Read the model definition and answer for the solid it produces. Units are mm, in the model's axes. A direction names the side the tool comes from. Give positions to 0.01 mm unless a question says otherwise; leave off trailing zeros. Order: outer loops, then holes, each group sorted by start corner. A loop starts at its lowest first (then second) coordinate and runs counter-clockwise, first axis right, second up.
Item 1: A cutting plane is placed at A-A (x = 50). Write down the section's boundary in (y, z), plus the area to 3 significant figures.
Item 2: A cutting plane is placed at C-C (z = 12). Write down the section's boundary in (x, y), plus the area to 3 significant figures.
Item 3: A cutting plane is placed at D-D (z = 15.5). Write down the section's boundary in (x, y).
Item 4: Which of the six approach directions +Z, -Z, +X, -X, +Y, -Y give full straight-line access (tool end or side, diameter ignored) to faces 4 (the face through (57.594, 9.126, 2.281)), 5 (the face through (32.1, 4.06, 29.14)), 6 (the face through (28.813, 2.958, 24.961)), 7 (the face through (1.2, 10.03, 12.95)), 8 (the face through (53, 13, 20))?
Item 5: A cutting plane is placed at B-B (y = 2.5). Write down the section's boundary in (x, z), plus the area to 3 significant figures.
Item 6: The mould has two halves that part along Z. Classify faces 1 (the face through (30, 6, 1)), 2 (the face through (2.281, 9.126, 2.406)), 3 (the face through (38.3, 8.6, 23)): +Z half, -Z half, draft (parallel to the pull), parting line (faces both ways), or undercut.
Item 7: Given pin 1 Ø3 at (x, z) = (28.5, 29) entering from +Y; pin 2 Ø8 at (y, z) = (9, 1.5) entering from -X; pin 3 Ø2 at (x, z) = (44.5, 26.5) entering from -Y; pin 4 Ø6 at (x, z) = (27.5, 15) entering from +Y, each flat-ended and moving along its own axis, determine where each tip first touches the part or whether it passes through.
Item 8: Find the intervals of material crossed by line 1 along Z through (x, y) = (30.2, 4.15); line 2 along X through (y, z) = (11.5, 18.5); line 3 along X through (y, z) = (16.5, 9), in increasing order.
from build123d import *

# Parameters (mm, degrees)
BOX_W           = 60
BOX_H           = 18
BOX_DEPTH       = 26
SKETCH003_R     = 7.7
POCKET_DEPTH    = 18.001
SKETCH004_R     = 1.4
POCKET001_DEPTH = 5
SKETCH002_R     = 1.5
POCKET002_DEPTH = 6
SKETCH005_R     = 1.4
POCKET003_DEPTH = 5
SKETCH017_W     = 13
SKETCH017_H     = 8
PAD_DEPTH       = 4
SKETCH018_W     = 9
SKETCH018_H     = 8
PAD001_DEPTH    = 4
SKETCH008_R     = 9.4
POCKET015_DEPTH = 34.001
FILLET_R        = 3
SKETCH007_R     = 1.45
SKETCH007_R_2   = 1.388343
POCKET016_DEPTH = 6
FILLET002_R     = 8


with BuildPart() as part:
    # Box → Box (new body)
    with BuildSketch(Plane.XY):
        with Locations((30, 9)):
            Rectangle(BOX_W, BOX_H)
    extrude(amount=BOX_DEPTH)

    # Sketch003 → Pocket (cut, through all)
    with BuildSketch(Plane(origin=(0, 18, 0), x_dir=(-1, 0, 0), z_dir=(0, 1, 0))):
        with Locations((-50, 12)):
            Circle(SKETCH003_R)
        with Locations((-10, 12)):
            Circle(SKETCH003_R)
    extrude(amount=-POCKET_DEPTH, mode=Mode.SUBTRACT)

    # Sketch004 → Pocket001 (cut)
    with BuildSketch(Plane.YZ.offset(60)):
        with Locations((9, 12)):
            Circle(SKETCH004_R)
    extrude(amount=-POCKET001_DEPTH, mode=Mode.SUBTRACT)

    # Sketch002 → Pocket002 (cut)
    with BuildSketch(Plane.XY.offset(26)):
        with Locations((39.5, 9.5)):
            Circle(SKETCH002_R)
        with Locations((53, 13)):
            Circle(SKETCH002_R)
    extrude(amount=-POCKET002_DEPTH, mode=Mode.SUBTRACT)

    # Sketch005 → Pocket003 (cut)
    with BuildSketch(Plane(origin=(0, 0, 0), x_dir=(0, -1, 0), z_dir=(-1, 0, 0))):
        with Locations((-9, 12)):
            Circle(SKETCH005_R)
    extrude(amount=-POCKET003_DEPTH, mode=Mode.SUBTRACT)

    # Sketch017 → Pad (new body)
    with BuildSketch(Plane(origin=(0, 0, 0), x_dir=(1, 0, 0), z_dir=(0, 0, -1))):
        with Locations((30.5, -4)):
            Rectangle(SKETCH017_W, SKETCH017_H)
    extrude(amount=PAD_DEPTH)

    # Sketch018 → Pad001 (new body)
    with BuildSketch(Plane.XY.offset(26)):
        with Locations((28.5, 4)):
            Rectangle(SKETCH018_W, SKETCH018_H)
    extrude(amount=PAD001_DEPTH)

    # Sketch008 → Pocket015 (cut, through all)
    with BuildSketch(Plane.XY.offset(30)):
        with Locations((28.2, 22.5)):
            Circle(SKETCH008_R)
    extrude(amount=-POCKET015_DEPTH, mode=Mode.SUBTRACT)

    # Fillet
    fillet_edges = [part.edges().sort_by_distance(p)[0] for p in [
        (24, 4, 30),
        (33, 4, 30),
        (37, 4, -4),
        (24, 4, -4),
    ]]
    fillet(fillet_edges, radius=FILLET_R)

    # Sketch007 → Pocket016 (cut)
    with BuildSketch(Plane.XZ):
        with Locations((30.2, 12.8)):
            Circle(SKETCH007_R)
        with Locations((30.2, 0.7)):
            Circle(SKETCH007_R)
        with Locations((30.2, 24.9)):
            Circle(SKETCH007_R_2)
    extrude(amount=-POCKET016_DEPTH, mode=Mode.SUBTRACT)

    # Fillet002
    fillet002_edges = [part.edges().sort_by_distance(p)[0] for p in [
        (0, 9, 26),
        (0, 9, 0),
        (60, 9, 0),
    ]]
    fillet(fillet002_edges, radius=FILLET002_R)


solid = part.part
Response values:
1. outline: (0, 0) - (18, 0) - (18, 4.3) - (0, 4.3) - close; (0, 19.7) - (18, 19.7) - (18, 26) - (0, 26) - close
1. area: 191 mm2
2. outline: (0, 0) - (2.3, 0) - (2.3, 7.6) - (0, 7.6) - close; (0, 10.4) - (2.3, 10.4) - (2.3, 18) - (0, 18) - close; (17.7, 0) - (28.99, 0) - (28.99, 6) - (31.41, 6) - (31.41, 0) - (42.3, 0) - (42.3, 18) - (36.45, 18) arc R9.4 cw to (19.95, 18) - (17.7, 18) - close; (57.7, 0) - (60, 0) - (60, 7.6) - (57.7, 7.6) - close; (57.7, 10.4) - (60, 10.4) - (60, 18) - (57.7, 18) - close
2. area: 441 mm2
3. outline: (0, 0) - (3.14, 0) - (3.14, 18) - (0, 18) - close; (16.86, 0) - (43.14, 0) - (43.14, 18) - (36.45, 18) arc R9.4 cw to (19.95, 18) - (16.86, 18) - close; (56.86, 0) - (60, 0) - (60, 18) - (56.86, 18) - close
4. face 4: -Z, +X, +Y, -Y
4. face 5: +Z, +X, +Y, -Y
4. face 6: -Y
4. face 7: -X
4. face 8: +Z
5. outline: (0, 8) arc R8 ccw to (8, 0) - (24, 0) - (24, -1) arc R3 ccw to (27, -4) - (34, -4) arc R3 ccw to (37, -1) - (37, 0) - (52, 0) arc R8 ccw to (60, 8) - (60, 26) - (33, 26) - (33, 27) arc R3 ccw to (30, 30) - (27, 30) arc R3 ccw to (24, 27) - (24, 26) - (8, 26) arc R8 ccw to (0, 18) - close; hole circle Ø15.4 at (10, 12); hole circle Ø2.9 at (30.2, 0.7); hole circle Ø2.9 at (30.2, 12.8); hole circle Ø2.78 at (30.2, 24.9); hole circle Ø15.4 at (50, 12)
5. area: 1,210 mm2
6. face 1: undercut
6. face 2: -Z half
6. face 3: draft
7. pin 1: stops at y = 8
7. pin 2: stops at x = 0.4
7. pin 3: stops at y = 0
7. pin 4: stops at y = 13.86
8. line 1: z = -4 to -0.75, 2.15 to 11.35, 14.25 to 23.51, 26.29 to 29.99
8. line 2: x = 0.02 to 5.87, 14.13 to 45.87, 54.13 to 60
8. line 3: x = 0 to 2.91, 17.09 to 20.96, 35.44 to 42.91, 57.09 to 60
